```python
from build123d import *

# Parameters (mm, degrees)
F1_DEPTH = 8
F2_DEPTH = 12.6
F4_DEPTH = 6.4


with BuildPart() as f1:
    # F0 (on Top) → F1 (new body)
    with BuildSketch(Plane.XY):
        Polygon((11.6008939222, -1.1197078275), (2, 11.0917733982), (2, -1.1197078275), align=None)
    extrude(amount=F1_DEPTH)

    # F0 (on Top) → F2 (join)
    with BuildSketch(Plane.XY):
        Polygon((0, 15.2802921725), (0, -10.1197078275), (2, -10.1197078275), (2, -3.1197078275), (15.4, -3.1197078275), (15.4, -1.1197078275), (11.6008939222, -1.1197078275), (2, -1.1197078275), (2, 11.0917733982), (2, 15.2802921725), align=None)
    extrude(amount=F2_DEPTH)

    # F3 (on face) → F4 (join)
    with BuildSketch(Plane(origin=(0, 0, 0), x_dir=(0, -1, 0), z_dir=(-1, 0, 0))):
        with BuildLine():
            ThreePointArc((0.299037522, 5.9791818809), (0.3145348993, 6.1392583384), (0.3197078275, 6.3))
            ThreePointArc((0.3197078275, 6.3), (0.3081127437, 6.5405015024), (0.2734350493, 6.7787720968))
            Line((0.2734350493, 6.7787720968), (-1.7932983009, 6.7125963443))
            Line((-1.7932983009, 6.7125963443), (-1.7676958282, 5.9130061284))
            Line((-1.7676958282, 5.9130061284), (0.299037522, 5.9791818809))
        make_face()
        with BuildLine():
            ThreePointArc((0.2734350493, 6.7787720968), (0.3081127437, 6.5405015024), (0.3197078275, 6.3))
            ThreePointArc((0.3197078275, 6.3), (0.3145348993, 6.1392583384), (0.299037522, 5.9791818809))
            Line((0.299037522, 5.9791818809), (1.1325090638, 6.0058692164))
            Line((1.1325090638, 6.0058692164), (1.1069065911, 6.8054594324))
            Line((1.1069065911, 6.8054594324), (0.2734350493, 6.7787720968))
        make_face()
        with BuildLine():
            Line((-1.7932983009, 6.7125963443), (0.2734350493, 6.7787720968))
            ThreePointArc((0.2734350493, 6.7787720968), (-0.4700047295, 8.123435456), (-1.8594740534, 8.7793296946))
            Line((-1.8594740534, 8.7793296946), (-1.7932983009, 6.7125963443))
        make_face()
        with BuildLine():
            ThreePointArc((-1.7015200757, 3.8462727781), (-0.3568567165, 4.589712557), (0.299037522, 5.9791818809))
            Line((0.299037522, 5.9791818809), (-1.7676958282, 5.9130061284))
            Line((-1.7676958282, 5.9130061284), (-1.7015200757, 3.8462727781))
        make_face()
        with BuildLine():
            Line((-1.7932983009, 6.7125963443), (-1.8594740534, 8.7793296946))
            ThreePointArc((-1.8594740534, 8.7793296946), (-2.2600924425, 8.7987260588), (-2.6586568197, 8.7538066885))
            Line((-2.6586568197, 8.7538066885), (-2.5924789427, 6.687006986))
            Line((-2.5924789427, 6.687006986), (-1.7932983009, 6.7125963443))
        make_face()
        with BuildLine():
            ThreePointArc((-2.6586568197, 8.7538066885), (-2.2600924425, 8.7987260588), (-1.8594740534, 8.7793296946))
            Line((-1.8594740534, 8.7793296946), (-1.8857514999, 9.6))
            Line((-1.8857514999, 9.6), (-2.6857514999, 9.6))
            Line((-2.6857514999, 9.6), (-2.6586568197, 8.7538066885))
        make_face()
        with BuildLine():
            Line((-1.6745311, 3.0033807187), (-1.7015200757, 3.8462727781))
            ThreePointArc((-1.7015200757, 3.8462727781), (-2.1000769886, 3.8012872265), (-2.5006985929, 3.8206170675))
            Line((-2.5006985929, 3.8206170675), (-2.4745311, 3.0033807187))
            Line((-2.4745311, 3.0033807187), (-1.6745311, 3.0033807187))
        make_face()
        with BuildLine():
            ThreePointArc((-2.5006985929, 3.8206170675), (-2.1000769886, 3.8012872265), (-1.7015200757, 3.8462727781))
            Line((-1.7015200757, 3.8462727781), (-1.7676958282, 5.9130061284))
            Line((-1.7676958282, 5.9130061284), (-2.56687647, 5.88741677))
            Line((-2.56687647, 5.88741677), (-2.5006985929, 3.8206170675))
        make_face()
        with BuildLine():
            Line((-2.5924789427, 6.687006986), (-2.6586568197, 8.7538066885))
            ThreePointArc((-2.6586568197, 8.7538066885), (-4.0035856251, 8.0104388285), (-4.6596218671, 6.6208181191))
            Line((-4.6596218671, 6.6208181191), (-2.5924789427, 6.687006986))
        make_face()
        with BuildLine():
            Line((-2.56687647, 5.88741677), (-2.5924789427, 6.687006986))
            Line((-2.5924789427, 6.687006986), (-4.6596218671, 6.6208181191))
            ThreePointArc((-4.6596218671, 6.6208181191), (-4.6790115973, 6.2199922728), (-4.6340193944, 5.8212279032))
            Line((-4.6340193944, 5.8212279032), (-2.56687647, 5.88741677))
        make_face()
        with BuildLine():
            ThreePointArc((-4.6340193944, 5.8212279032), (-3.8904282184, 4.4764225531), (-2.5006985929, 3.8206170675))
            Line((-2.5006985929, 3.8206170675), (-2.56687647, 5.88741677))
            Line((-2.56687647, 5.88741677), (-4.6340193944, 5.8212279032))
        make_face()
        with BuildLine():
            ThreePointArc((-4.6340193944, 5.8212279032), (-4.6790115973, 6.2199922728), (-4.6596218671, 6.6208181191))
            Line((-4.6596218671, 6.6208181191), (-5.4930934089, 6.5941307836))
            Line((-5.4930934089, 6.5941307836), (-5.4674909362, 5.7945405676))
            Line((-5.4674909362, 5.7945405676), (-4.6340193944, 5.8212279032))
        make_face()
    extrude(amount=F4_DEPTH)


solid = f1.part
```
Could you check a few things on this model? Use its own coordinates, in mm. A direction names the side the tool comes from. Coordinates: 2 decimals unless noted, no trailing zeros. Write each loop counter-clockwise with the first axis right and the second up, starting at its lowest first coordinate (ties: lowest second). Pieces come first, ordered by that corner, then holes. Notation, with made-up numbers: (16, -39) - (31, -39) arc R32 ccw to (31, -6) - close; hole circle Ø1 at (-33, 64.25). An arc over 180 degrees is marked (long way). Use a Markdown table: item, result.
Q1. Please list where these lines run through material, in increasing order: L1, parallel to X at y = 0.5, z = 11.25; L2, parallel to X at y = -3, z = 9.25; L3, parallel to Y at x = 12.75, z = 11.5.
Geometry check:
| item | result |
|---|---|
| L1 | x = 0 to 2 |
| L2 | x = 0 to 15.4 |
| L3 | y = -3.12 to -1.12 |
Q2. Imagine slicing it at B-B (z = 2). List the corners of the cut face in (x, y) for me.
Geometry check:
| item | result |
|---|---|
| outline | (0, -10.12) - (2, -10.12) - (2, -3.12) - (15.4, -3.12) - (15.4, -1.12) - (11.6, -1.12) - (2, 11.09) - (2, 15.28) - (0, 15.28) - close |
Q3. Imagine slicing it at A-A (x = -3.75). List the corners of the cut face in (y, z) for me.
Geometry check:
| item | result |
|---|---|
| outline | (-1.13, 6.01) - (-0.3, 5.98) arc R2.5 ccw to (1.7, 3.85) - (1.67, 3) - (2.47, 3) - (2.5, 3.82) arc R2.5 ccw to (4.63, 5.82) - (5.47, 5.79) - (5.49, 6.59) - (4.66, 6.62) arc R2.5 ccw to (2.66, 8.75) - (2.69, 9.6) - (1.89, 9.6) - (1.86, 8.78) arc R2.5 ccw to (-0.27, 6.78) - (-1.11, 6.81) - close; hole (1.77, 5.91) - (2.57, 5.89) - (2.59, 6.69) - (1.79, 6.71) - close |
Q4. I'm going to push flat-ended pins straight in: pin 1 Ø6.5 at (y, z) = (6.5, 4) entering from +X; pin 2 Ø5.5 at (y, z) = (-6, 5) entering from +X; pin 3 Ø6 at (x, z) = (12, 2) entering from -Y. Where does each tip first touch, or does it pass through?
Geometry check:
| item | result |
|---|---|
| pin 1 | stops at x = 8.17 |
| pin 2 | stops at x = 2 |
| pin 3 | stops at y = -3.12 |
Q5. Imagine slicing it at D-D (x = 12). List the corners of the cut face in (y, z) for me, and give its area (3 significant figures).
Geometry check:
| item | result |
|---|---|
| outline | (-3.12, 0) - (-1.12, 0) - (-1.12, 12.6) - (-3.12, 12.6) - close |
| area | 25.2 mm2 |
Q6. Which directions (+Z, -Z, +X, -X, +Y, -Y) give clear straight access to the entire face, cutting with the end or side of a thin tool? Please do faces 1 (the flat face through (4, 0, 0)), 2 (the flat face through (2, -7, 6)), 3 (the flat face through (2, 9, 9)).
Geometry check:
| item | result |
|---|---|
| face 1 | -Z, +X, -X, +Y, -Y |
| face 2 | +Z, -Z, +X, -Y |
| face 3 | +Z, +X, +Y |
Q7. Imagine slicing it at C-C (y = 5). List the corners of the cut face in (x, z) for me.
Geometry check:
| item | result |
|---|---|
| outline | (-6.4, 5.81) - (0, 5.81) - (0, 0) - (6.79, 0) - (6.79, 8) - (2, 8) - (2, 12.6) - (0, 12.6) - (0, 6.61) - (-6.4, 6.61) - close |
Q8. Thinking about a two-plate mould opening in Y: for faces 4 (the flat face through (9, -3.12, 6)), 5 (the flat face through (0, 2.2, 6.3)), 6 (the flat face through (10, -1.12, 9)), 7 (the flat face through (4, -2, 12.6)), which applies, +Y half, -Y half, draft (parallel to the pull), parting line (faces both ways), or undercut?
Geometry check:
| item | result |
|---|---|
| face 4 | -Y half |
| face 5 | undercut |
| face 6 | +Y half |
| face 7 | draft |
